Part model, mm, in its own coordinate system. A direction names the side the tool comes from. Round coordinates to 2 decimals unless told otherwise and drop trailing zeros. Write each loop counter-clockwise with the first axis right and the second up, starting at its lowest first coordinate (ties: lowest second). Pieces come first, ordered by that corner, then holes. Notation, with made-up numbers: M 21,10 L 76,10 A15 ccw 76,31 Z; hole C 25,78.25 d10. An arc over 180 degrees is marked long. Answer as a JSON object with one key per item and string values. Group by question number.
1. Band-saw the part on D-D, the plane x = 14. Write the cut outline in (y, z), plus the area to 3 significant figures.
2. Band-saw the part on B-B, the plane y = 0. Write the cut outline in (x, z).
3. Band-saw the part on A-A, the plane x = -5. Write the cut outline in (y, z).
4. Two-plate mould, pull along Y, no slides. Class faces 1 (the face through (9, -4, 1)), 2 (the face through (-18.986, 0.616, 0.493)), 3 (the face through (-21.987, 0.652, 0.493)): +Y half, -Y half, draft (parallel to the pull), parting line (faces both ways), or undercut.
5. Band-saw the part on C-C, the plane z = 0.65. Write the cut outline in (x, y).
6. Which spindle directions (+Z, -Z, +X, -X, +Y, -Y) get a long thin tool onto all of the face, cutting with end or side? Do faces 4 (the face through (19.5, -6.642, 0.5)), 5 (the face through (9, -4, 0)), 6 (the face through (19.8, 6.642, 0.5)). Say none if no direction does.
7. Drill centre lines: line 1 (Y direction, x = -5, z = 0.35); line 2 (X direction, y = 0, z = 0.2); line 3 (Y direction, x = 25.5, z = 0.95). Where is each one in solid material? Low to high. Write a range as from..to.
8. Drop flat-ended pins along their axis: pin 1 (1 mm diameter, centred on x = 20.5, y = 4, fed in from -Z); pin 2 (0.5 mm diameter, centred on x = 21.5, z = 0.5, fed in from -Y); pin 3 (0.5 mm diameter, centred on x = 23.5, z = 0.5, fed in from +Y). Give the stop position or say it passes through.
from build123d import *

# Parameters (mm, degrees)
PAD_DEPTH    = 1
SKETCH_R     = 14
POCKET_DEPTH = 1.001


with BuildPart() as part:
    # Sketch004 → Pad (new body)
    with BuildSketch(Plane.XY):
        with BuildLine():
            Line((28.648583, 6.642429), (10.648583, 6.642429))
            ThreePointArc((10.648583, 6.642429), (-22, 0), (10.648583, -6.642429))
            Line((10.648583, -6.642429), (28.648583, -6.642429))
            Line((28.648583, 0), (28.648583, -6.642429))
            Line((28.648583, 6.642429), (28.648583, 0))
        make_face()
    extrude(amount=PAD_DEPTH)

    # Sketch → Pocket (cut, through all)
    with BuildSketch(Plane.XY):
        with Locations((-5, 0)):
            Circle(SKETCH_R)
    extrude(amount=POCKET_DEPTH, mode=Mode.SUBTRACT)


solid = part.part
Worked answers:
{
 "1": {"outline": "M -6.64,0 L 6.64,0 L 6.64,1 L -6.64,1 Z", "area": "13.3 mm^2"},
 "2": {"outline": "M -22,0 L -19,0 L -19,1 L -22,1 Z; M 9,0 L 28.65,0 L 28.65,1 L 9,1 Z"},
 "3": {"outline": "M -17,0 L -14,0 L -14,1 L -17,1 Z; M 14,0 L 17,0 L 17,1 L 14,1 Z"},
 "4": {"face 1": "draft", "face 2": "undercut", "face 3": "parting line"},
 "5": {"outline": "M 10.65,-6.64 L 28.65,-6.64 L 28.65,6.64 L 10.65,6.64 A17 ccw long Z; hole C -5,0 d28"},
 "6": {"face 4": "+Z, -Z, +X, -Y", "face 5": "-Z, +X, -X, +Y, -Y", "face 6": "+Z, -Z, +X, +Y"},
 "7": {"line 1": "y = -17..-14, 14..17", "line 2": "x = -22..-19, 9..28.65", "line 3": "y = -6.64..6.64"},
 "8": {"pin 1": "stops at z = 0", "pin 2": "stops at y = -6.64", "pin 3": "stops at y = 6.64"}
}
